Here's how the part is built. I have some questions about the finished solid (model axes, mm). Round coordinates to 2 decimals unless told otherwise and drop trailing zeros. Write each loop counter-clockwise with the first axis right and the second up, starting at its lowest first coordinate (ties: lowest second). Pieces come first, ordered by that corner, then holes. Notation, with made-up numbers: M 7.5,58 L 56.5,58 A19 ccw 56.5,70 Z; hole C 14.5,88 d3. An arc over 180 degrees is marked long. Use a Markdown table: item, result. Add a question column.
```python
from build123d import *

# Parameters (mm, degrees)
SKETCH1_W           = 54
SKETCH1_H           = 54
SKETCH1_R           = 3
BOSS_EXTRUDE1_DEPTH = 10


with BuildPart() as part:
    # Sketch1 → Boss-Extrude1 (new body)
    with BuildSketch(Plane(origin=(0, 0, 0), x_dir=(1, 0, 0), z_dir=(0, 1, 0))):
        Rectangle(SKETCH1_W, SKETCH1_H)
        with Locations((-18, -18)):
            Circle(SKETCH1_R, mode=Mode.SUBTRACT)
        with Locations((0, -18)):
            Circle(SKETCH1_R, mode=Mode.SUBTRACT)
        with Locations((18, -18)):
            Circle(SKETCH1_R, mode=Mode.SUBTRACT)
        with Locations((18, 0)):
            Circle(SKETCH1_R, mode=Mode.SUBTRACT)
        with Locations((18, 18)):
            Circle(SKETCH1_R, mode=Mode.SUBTRACT)
        with Locations((0, 18)):
            Circle(SKETCH1_R, mode=Mode.SUBTRACT)
        with Locations((-18, 18)):
            Circle(SKETCH1_R, mode=Mode.SUBTRACT)
        with Locations((-18, 0)):
            Circle(SKETCH1_R, mode=Mode.SUBTRACT)
        Circle(SKETCH1_R, mode=Mode.SUBTRACT)
    extrude(amount=BOSS_EXTRUDE1_DEPTH)


solid = part.part
```
Item 1: I need wall thicknesses on probe 1 along Z at (x, y) = (0, 3); probe 2 along X at (y, z) = (2.75, 20). Which ranges of each line are inside material? Lowest first, please. Write a range as from..to.
Item 2: Imagine slicing it at A-A on z = -18. List the corners of the cut face in (x, y) for me, plus the area to 3 significant figures.
Item 3: For pin 1 Ø9.5 at (x, z) = (18, 18) entering from +Y; pin 2 Ø5.5 at (x, z) = (0, 18) entering from +Y, each with a flat end and sliding along its axis, tell me the tip position at first contact or that it passes through.
Item 4: If we mould it in two halves opening along Z, with no side actions, what happens to faces 1 (the face through (-3, 5, 0)), 2 (the face through (6, 0, 0)), 3 (the face through (0, 5, 27))? For each: +Z half, -Z half, draft (parallel to the pull), parting line (faces both ways), or undercut.
Item 5: Imagine slicing it at B-B on x = 0. List the corners of the cut face in (y, z) for me.
Item 6: Imagine slicing it at C-C on y = 7.5. Count the separate pieces of the cut face and the enclosed holes in it, plus the area to 3 significant figures.
The answers:
| question | item | result |
|---|---|---|
| 1 | probe 1 | -27..-21, -15..-3, 3..15, 21..27 |
| 1 | probe 2 | -27..-20.24, -15.76..-2.24, 2.24..15.76, 20.24..27 |
| 2 | outline | M -27,0 L -21,0 L -21,10 L -27,10 Z; M -15,0 L -3,0 L -3,10 L -15,10 Z; M 3,0 L 15,0 L 15,10 L 3,10 Z; M 21,0 L 27,0 L 27,10 L 21,10 Z |
| 2 | area | 360 mm² |
| 3 | pin 1 | y = 10 |
| 3 | pin 2 | through |
| 4 | face 1 | undercut |
| 4 | face 2 | draft |
| 4 | face 3 | +Z half |
| 5 | outline | M 0,-27 L 10,-27 L 10,-21 L 0,-21 Z; M 0,-15 L 10,-15 L 10,-3 L 0,-3 Z; M 0,3 L 10,3 L 10,15 L 0,15 Z; M 0,21 L 10,21 L 10,27 L 0,27 Z |
| 6 | separate pieces | 1 |
| 6 | enclosed holes | 9 |
| 6 | area | 2,660 mm² |
